```python
from build123d import *

# Parameters (mm, degrees)
F0_R      = 1.75
F1_DEPTH  = 7
F2_W      = 14
F2_H      = 44
F2_R      = 1.75
F3_DEPTH  = 15
F4_R      = 2.5
F4_R_2    = 1.75
F5_DEPTH  = 25
F6_R      = 4
F7_DEPTH  = 2
F8_W      = 14
F8_H      = 32
F9_DEPTH  = 10
F10_W     = 14
F10_H     = 32
F11_DEPTH = 10
F12_R     = 1.75
F13_DEPTH = 25
F14_SIZE  = 10


with BuildPart() as f1:
    # F0 (on Front) → F1 (new body)
    with BuildSketch(Plane.XZ):
        with BuildLine():
            Line((0, 44), (0, 0))
            Line((0, 0), (14, 0))
            Line((14, 0), (14, 13.055728))
            ThreePointArc((14, 13.055728), (22, 34), (30, 13.055728))
            Line((30, 13.055728), (30, 0))
            Line((30, 0), (44, 0))
            Line((44, 0), (44, 44))
            Line((44, 44), (0, 44))
        make_face()
        with Locations((6.5, 6.5)):
            Circle(F0_R, mode=Mode.SUBTRACT)
        with Locations((37.5, 6.5)):
            Circle(F0_R, mode=Mode.SUBTRACT)
        with Locations((6.5, 37.5)):
            Circle(F0_R, mode=Mode.SUBTRACT)
        with Locations((37.5, 37.5)):
            Circle(F0_R, mode=Mode.SUBTRACT)
    extrude(amount=F1_DEPTH)

    # F2 (on face) → F3 (join)
    with BuildSketch(Plane.XZ.offset(7)):
        with Locations((7, 22)):
            Rectangle(F2_W, F2_H)
        with Locations((6.5, 6.5)):
            Circle(F2_R, mode=Mode.SUBTRACT)
        with Locations((6.5, 37.5)):
            Circle(F2_R, mode=Mode.SUBTRACT)
    extrude(amount=F3_DEPTH)

    # F4 (on face) → F5 (cut)
    with BuildSketch(Plane.YZ.offset(14)):
        with Locations((-14.5, 26)):
            Circle(F4_R)
        with Locations((-14.5, 6)):
            Circle(F4_R_2)
    extrude(amount=-F5_DEPTH, mode=Mode.SUBTRACT)

    # F6 (on face) → F7 (cut)
    with BuildSketch(Plane.YZ.offset(14)):
        with Locations((-14.5, 6)):
            Circle(F6_R)
    extrude(amount=-F7_DEPTH, mode=Mode.SUBTRACT)

    # F8 (on face) → F9 (join)
    with BuildSketch(Plane.XY.offset(44)):
        with Locations((7, -6)):
            Rectangle(F8_W, F8_H)
    extrude(amount=F9_DEPTH)

    # F10 (on face) → F11 (join)
    with BuildSketch(Plane(origin=(0, 0, 0), x_dir=(1, 0, 0), z_dir=(0, 0, -1))):
        with Locations((7, 6)):
            Rectangle(F10_W, F10_H)
    extrude(amount=F11_DEPTH)

    # F12 (on face) → F13 (cut)
    with BuildSketch(Plane.YZ.offset(14)):
        with Locations((0, 49)):
            Circle(F12_R)
        with Locations((0, -5)):
            Circle(F12_R)
    extrude(amount=-F13_DEPTH, mode=Mode.SUBTRACT)

    # F14
    f14_edges = [f1.edges().sort_by_distance(p)[0] for p in [
        (7, -22, 54),
        (7, -22, -10),
    ]]
    chamfer(f14_edges, length=F14_SIZE)


solid = f1.part
```
Geometry check sheet. Reference: the model listing, model coordinates, mm. A direction names the side the tool comes from. Give positions to 0.01 mm unless a question says otherwise; leave off trailing zeros. Loops run counter-clockwise (first coordinate to the right, second up) from the corner with the lowest first, then second, coordinate; pieces in that order, holes last. Notation, with made-up numbers: M -14,20 L 31,20 A21 ccw 31,53 Z; hole C 62,-31.75 d2. An arc over 180 degrees is marked long. Answer as CSV lines item,"result".
Item 1: Cross-section at D-D on z = 49. Record the cut outline in (x, y), and give its area (3 significant figures).
Values:
outline,"M 0,-17 L 14,-17 L 14,-1.75 L 0,-1.75 Z; M 0,1.75 L 14,1.75 L 14,10 L 0,10 Z"
area,"329 mm²"
Item 2: Cross-section at C-C on x = 37.5. Record the cut outline in (y, z).
Values:
outline,"M -7,0 L 0,0 L 0,4.75 L -7,4.75 Z; M -7,8.25 L 0,8.25 L 0,35.75 L -7,35.75 Z; M -7,39.25 L 0,39.25 L 0,44 L -7,44 Z"
Item 3: Depth check by flat-ended pin: P1, Ø5.5, axis at x = 6.5, z = 37.5, coming from the +Y side; P2, Ø5, axis at x = 39, y = -8.5, coming from the +Z side; P3, Ø3.5, axis at x = 37.5, y = -4.5, coming from the -Z side. Enter the tip coordinate at first touch or a pass-through.
Values:
P1,"stops at y = 0"
P2,"stops at z = 44"
P3,"stops at z = 0"
Item 4: Cross-section at A-A on y = 5. Record the cut outline in (x, z), and give its area (3 significant figures).
Values:
outline,"M 0,-10 L 14,-10 L 14,0 L 0,0 Z; M 0,44 L 14,44 L 14,54 L 0,54 Z"
area,"280 mm²"
Item 5: Access from +Z, -Z, +X, -X, +Y, -Y to the whole of each face (thin tool, end or side, straight path). Record for faces 4 (the flat face through (7, 5, 0)), 5 (the cylindrical face through (22, -3, 34)), 6 (the flat face through (30, -3, 7)), 7 (the flat face through (37, -3, 0)).
Values:
face 4,"+X, -X, +Y"
face 5,"+Y"
face 6,"-Z, +Y, -Y"
face 7,"-Z, +X, +Y, -Y"
Item 6: Cross-section at B-B on z = 37.5. Record the cut outline in (x, y), and give its area (4 significant figures).
Values:
outline,"M 0,-22 L 4.75,-22 L 4.75,0 L 0,0 Z; M 8.25,-22 L 14,-22 L 14,-7 L 35.75,-7 L 35.75,0 L 8.25,0 Z; M 39.25,-7 L 44,-7 L 44,0 L 39.25,0 Z"
area,"416.5 mm²"
Item 7: Release check for a two-part mould opening along Z. For faces 1 (the cylindrical face through (13, -17.7, 3.6)), 2 (the flat face through (7, -17, 49)), 3 (the flat face through (44, -3, 22)) record: pulls with the +Z half, pulls with the -Z half, needs draft (parallel to the pull), parting line crosses it, or undercut.
Values:
face 1,"undercut"
face 2,"pulls with the +Z half"
face 3,"needs draft"
Item 8: Material ranges on line 1 (Y direction, x = 3, z = 6); line 2 (X direction, y = -10.75, z = 6.5); line 3 (X direction, y = -4.5, z = 10), recorded low to high.
Values:
line 1,"y = -22 to -16.25, -12.75 to 0"
line 2,"x = 0 to 4.75, 8.25 to 12"
line 3,"x = 0 to 14, 30 to 44"
